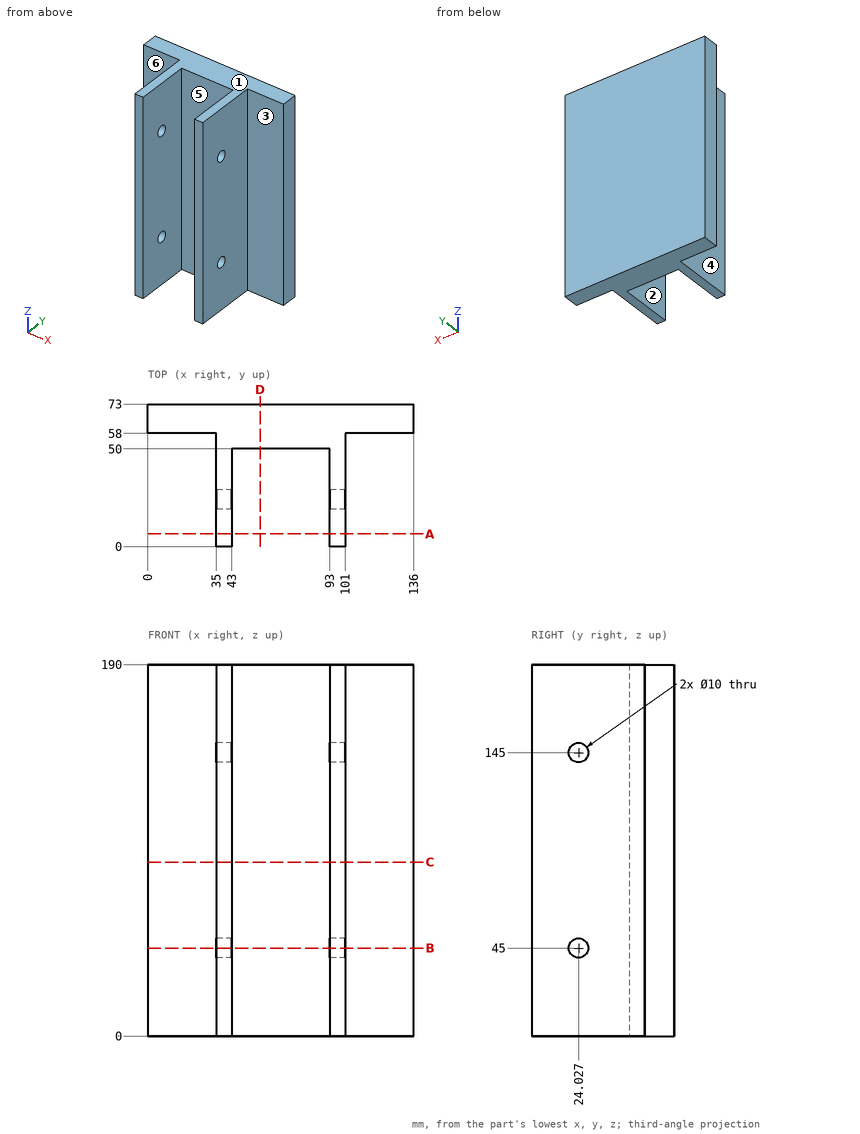
Design review of the part shown in the three views and the two pictorial views. Dimensions are in mm from the part's minimum x, y and z. A direction names the side the tool comes from. Round coordinates to 2 decimals unless told otherwise and drop trailing zeros. Write each loop counter-clockwise with the first axis right and the second up, starting at its lowest first coordinate (ties: lowest second). Pieces come first, ordered by that corner, then holes. Notation, with made-up numbers: (61, -36) - (101, -36) arc R33 ccw to (101, 2) - close; hole circle Ø2 at (40.5, -23.75). An arc over 180 degrees is marked (long way). Answer as CSV lines item,"result". Start each with the question number.
(1) Machinability: for the marked faces 1, 2 and 3, which of the approach directions +Z, -Z, +X, -X, +Y, -Y give a long, thin tool a straight path to every point of the face, cutting with its end or side? Answer none if there is none.
(2) Add section C-C, the plane z = 89. State the section outline as (x, y) points, plus the area to 3 significant figures.
(3) For pin 1 (17.5 mm diameter, centred on x = 20, z = 52, fed in from -Y); pin 2 (9 mm diameter, centred on y = 24.03, z = 145, fed in from +X); pin 3 (11.5 mm diameter, centred on y = 24.03, z = 145, fed in from -X); pin 4 (6 mm diameter, centred on y = 30, z = 162, fed in from +X), all flat-tipped, find the tip position at first contact; note any pin that passes through.
(4) Add section D-D, the plane x = 57.5. State the section outline as (y, z) points, plus the area to 3 significant figures.
(5) Add section A-A, the plane y = 6.5. State the section outline as (x, z) points.
(6) Add section B-B, the plane z = 45. State the section outline as (x, y) points.
(7) Mouldability with a two-part tool opening along X and no side actions: class the marked faces 4, 5 and 6 as +X half, -X half, draft (parallel to the pull), parting line (faces both ways), or undercut.
(8) For line 1 (X direction, y = 32.5, z = 90); line 2 (Y direction, x = 97, z = 45); line 3 (Y direction, x = 80, z = 172.5), list the stretches that pass through material, from the lowest coordinate up.
From the geometry:
1,face 1,"+Z, +X, -X, +Y, -Y"
1,face 2,"+Z, -Z, -Y"
1,face 3,"+Z, -Z, +X, -Y"
2,outline,"(0, 58) - (35, 58) - (35, 0) - (43, 0) - (43, 50) - (93, 50) - (93, 0) - (101, 0) - (101, 58) - (136, 58) - (136, 73) - (0, 73) - close"
2,area,"3,370 mm²"
3,pin 1,"stops at y = 58"
3,pin 2,"passes through"
3,pin 3,"stops at x = 35"
3,pin 4,"stops at x = 101"
4,outline,"(50, 0) - (73, 0) - (73, 190) - (50, 190) - close"
4,area,"4,370 mm²"
5,outline,"(35, 0) - (43, 0) - (43, 190) - (35, 190) - close; (93, 0) - (101, 0) - (101, 190) - (93, 190) - close"
6,outline,"(0, 58) - (35, 58) - (35, 29.03) - (43, 29.03) - (43, 50) - (93, 50) - (93, 29.03) - (101, 29.03) - (101, 58) - (136, 58) - (136, 73) - (0, 73) - close; (35, 0) - (43, 0) - (43, 19.03) - (35, 19.03) - close; (93, 0) - (101, 0) - (101, 19.03) - (93, 19.03) - close"
7,face 4,"-X half"
7,face 5,"undercut"
7,face 6,"draft"
8,line 1,"x = 35 to 43, 93 to 101"
8,line 2,"y = 0 to 19.03, 29.03 to 73"
8,line 3,"y = 50 to 73"
